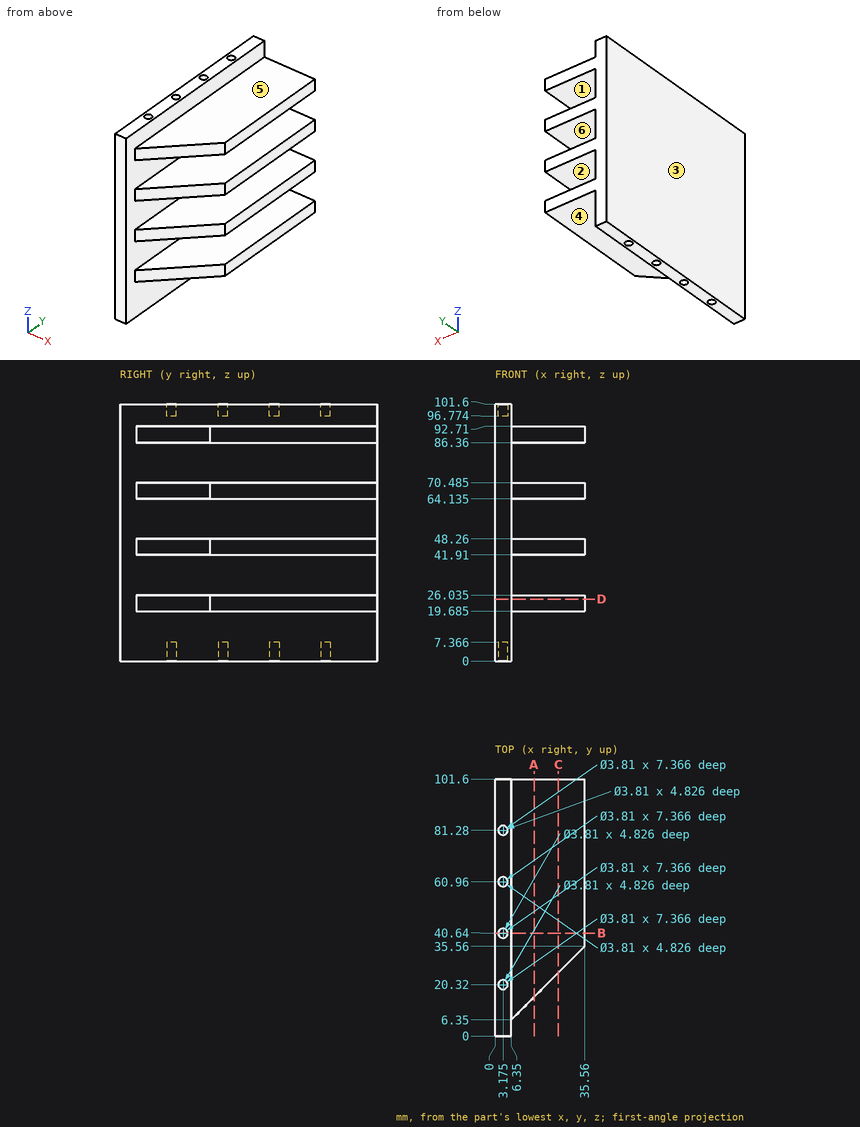
Answer from the drawing. Dimensions are ordinates in mm from the lowest x, y and z of the part. A direction names the side the tool comes from. Coordinates: 2 decimals unless noted, no trailing zeros. Loops run counter-clockwise (first coordinate to the right, second up) from the corner with the lowest first, then second, coordinate; pieces in that order, holes last.
1) Consider probe 1 along Z at (x, y) = (19.5, 65.5) (3 decimals); probe 2 along X at (y, z) = (8, 63); probe 3 along Y at (x, z) = (22.5, 69). Determine where each line is inside the solid, lowest interval first.
Results:
probe 1: z = 19.685 to 26.035, 41.91 to 48.26, 64.135 to 70.485, 86.36 to 92.71
probe 2: x = 0 to 6.35
probe 3: y = 22.5 to 101.6
2) Section A-A (x = 15.5) is taken. Give the vertices of the cut face in (y, z) (3 decimals).
Results:
outline: (15.5, 19.685) - (101.6, 19.685) - (101.6, 26.035) - (15.5, 26.035) - close; (15.5, 41.91) - (101.6, 41.91) - (101.6, 48.26) - (15.5, 48.26) - close; (15.5, 64.135) - (101.6, 64.135) - (101.6, 70.485) - (15.5, 70.485) - close; (15.5, 86.36) - (101.6, 86.36) - (101.6, 92.71) - (15.5, 92.71) - close
3) Flat-ended cylindrical pins translate along their axes: pin 1 (6 mm diameter, centred on x = 3.175, y = 20.32, fed in from +Z); pin 2 (2.5 mm diameter, centred on x = 3.175, y = 60.96, fed in from +Z); pin 3 (6 mm diameter, centred on x = 18, y = 56, fed in from -Z) (3 decimals); pin 4 (1.9 mm diameter, centred on x = 3, y = 21, fed in from -Z). Find the tip coordinate at first contact, or state that the pin passes through.
Results:
pin 1: stops at z = 101.6
pin 2: stops at z = 96.77
pin 3: stops at z = 19.685
pin 4: stops at z = 7.37
4) Section B-B (y = 40.64) is taken. Give the vertices of the cut face in (x, z) (3 decimals).
Results:
outline: (0, 0) - (1.27, 0) - (1.27, 7.366) - (5.08, 7.366) - (5.08, 0) - (6.35, 0) - (6.35, 19.685) - (35.56, 19.685) - (35.56, 26.035) - (6.35, 26.035) - (6.35, 41.91) - (35.56, 41.91) - (35.56, 48.26) - (6.35, 48.26) - (6.35, 64.135) - (35.56, 64.135) - (35.56, 70.485) - (6.35, 70.485) - (6.35, 86.36) - (35.56, 86.36) - (35.56, 92.71) - (6.35, 92.71) - (6.35, 101.6) - (5.08, 101.6) - (5.08, 96.774) - (1.27, 96.774) - (1.27, 101.6) - (0, 101.6) - close
5) Section D-D (z = 24.5) is taken. Give the vertices of the cut face in (x, y).
Results:
outline: (0, 0) - (6.35, 0) - (6.35, 6.35) - (35.56, 35.56) - (35.56, 101.6) - (0, 101.6) - close
6) For a pull along Z with two mould halves and no side action, classify the marked faces 1, 2, 3 and 4 as +Z half, -Z half, draft (parallel to the pull), parting line (faces both ways), or undercut.
Results:
face 1: undercut
face 2: undercut
face 3: draft
face 4: -Z half
7) For the marked faces 5 and 6, determine the directions among +Z, -Z, +X, -X, +Y, -Y from which every point of the face is accessible in a straight line to the end or side of a thin tool.
Results:
face 5: +Z, +X, +Y, -Y
face 6: +X, +Y, -Y
8) Section C-C (x = 25) is taken. Give the vertices of the cut face in (y, z) (3 decimals).
Results:
outline: (25, 19.685) - (101.6, 19.685) - (101.6, 26.035) - (25, 26.035) - close; (25, 41.91) - (101.6, 41.91) - (101.6, 48.26) - (25, 48.26) - close; (25, 64.135) - (101.6, 64.135) - (101.6, 70.485) - (25, 70.485) - close; (25, 86.36) - (101.6, 86.36) - (101.6, 92.71) - (25, 92.71) - close
